```python
from build123d import *

# Parameters (mm, degrees)
F0_R     = 1
F1_DEPTH = 75
F2_W     = 65
F2_H     = 95
F3_DEPTH = 63
F4_R     = 1.7
F5_DEPTH = 7.001
F6_R     = 4


with BuildPart() as f1:
    # F0 (on Right) → F1 (new body)
    with BuildSketch(Plane.YZ):
        with BuildLine():
            Line((0, 72), (0, 0))
            Line((0, 0), (50, 0))
            ThreePointArc((50, 0), (64.142136, 5.857864), (70, 20))
            Line((70, 20), (70, 69))
            ThreePointArc((70, 69), (69.12132, 71.12132), (67, 72))
            Line((67, 72), (60.95857, 72))
            ThreePointArc((60.95857, 72), (57.269006, 70.731503), (55.139509, 67.462372))
            Line((55.139509, 67.462372), (50.118783, 47.483938))
            ThreePointArc((50.118783, 47.483938), (49.969332, 46.149869), (50.180201, 44.824121))
            Line((50.180201, 44.824121), (53.069629, 35.224997))
            ThreePointArc((53.069629, 35.224997), (50.230854, 29.932138), (44.933914, 32.763293))
            Line((44.933914, 32.763293), (41.069777, 45.467928))
            ThreePointArc((41.069777, 45.467928), (40.854911, 46.800259), (41.00419, 48.141522))
            Line((41.00419, 48.141522), (45.437209, 65.781356))
            ThreePointArc((45.437209, 65.781356), (44.530911, 70.074637), (40.587992, 72))
            Line((40.587992, 72), (0, 72))
        make_face()
        with Locations((66, 68)):
            Circle(F0_R, mode=Mode.SUBTRACT)
    extrude(amount=F1_DEPTH)

    # F2 (on face) → F3 (cut)
    with BuildSketch(Plane(origin=(0, 70, 0), x_dir=(-1, 0, 0), z_dir=(0, 1, 0))):
        with Locations((-37.5, 41.631669)):
            Rectangle(F2_W, F2_H)
    extrude(amount=-F3_DEPTH, mode=Mode.SUBTRACT)

    # F4 (on face) → F5 (cut, through all)
    with BuildSketch(Plane(origin=(0, 7, 0), x_dir=(-1, 0, 0), z_dir=(0, 1, 0))):
        with Locations((-61.5, 60)):
            Circle(F4_R)
        with Locations((-61.5, 12)):
            Circle(F4_R)
        with Locations((-13.5, 12)):
            Circle(F4_R)
        with Locations((-13.5, 60)):
            Circle(F4_R)
        with Locations((-37.5, 52)):
            Circle(F4_R)
        with Locations((-37.5, 20)):
            Circle(F4_R)
    extrude(amount=-F5_DEPTH, mode=Mode.SUBTRACT)

    # F6
    f6_edges = [f1.edges().sort_by_distance(p)[0] for p in [
        (70, 7, 36),
        (5, 7, 36),
    ]]
    fillet(f6_edges, radius=F6_R)


solid = f1.part
```
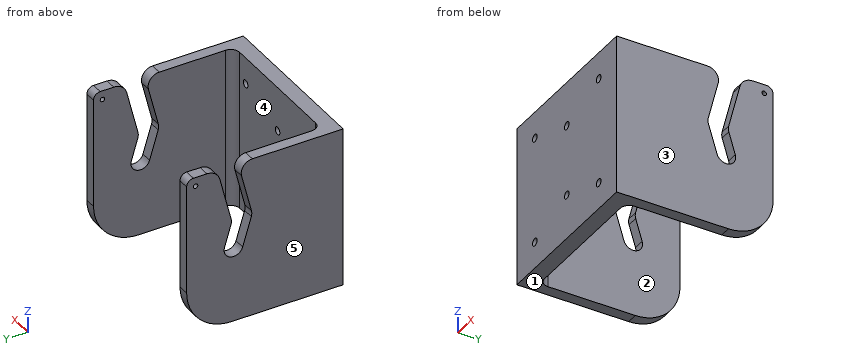
Work out the finished part from the listing and answer in its coordinate system (mm). Face numbers are marked on the shaded views. A direction names the side the tool comes from. Give positions to 0.01 mm unless a question says otherwise; leave off trailing zeros. Write each loop counter-clockwise with the first axis right and the second up, starting at its lowest first coordinate (ties: lowest second). Pieces come first, ordered by that corner, then holes.
(1) Which of the six approach directions +Z, -Z, +X, -X, +Y, -Y give full straight-line access (tool end or side, diameter ignored) to the marked faces 1 and 2?
Final values:
face 1: -Z, +X, -X, +Y, -Y
face 2: +Z, -Z, +Y
(2) The part is cut by section A-A on y = 20. Write down the section's boundary in (x, z).
Final values:
outline: (0, 0) - (5, 0) - (5, 72) - (0, 72) - close; (70, 0) - (75, 0) - (75, 72) - (70, 72) - close
(3) The part is cut by section D-D on z = 34. Write down the section's boundary in (x, y), plus the area to 3 significant figures.
Final values:
outline: (0, 0) - (75, 0) - (75, 44.56) - (70, 44.56) - (70, 11) arc R4 cw to (66, 7) - (9, 7) arc R4 cw to (5, 11) - (5, 44.56) - (0, 44.56) - close; (0, 53.25) - (5, 53.25) - (5, 70) - (0, 70) - close; (70, 53.25) - (75, 53.25) - (75, 70) - (70, 70) - close
area: 1,070 mm2
(4) The part is cut by section C-C on z = 23.5. Write down the section's boundary in (x, y).
Final values:
outline: (0, 0) - (75, 0) - (75, 70) - (70, 70) - (70, 11) arc R4 cw to (66, 7) - (9, 7) arc R4 cw to (5, 11) - (5, 70) - (0, 70) - close
(5) The part is cut by section B-B on x = 37.5. Write down the section's boundary in (y, z).
Final values:
outline: (0, 0) - (7, 0) - (7, 18.3) - (0, 18.3) - close; (0, 21.7) - (7, 21.7) - (7, 50.3) - (0, 50.3) - close; (0, 53.7) - (7, 53.7) - (7, 72) - (0, 72) - close
(6) Straight lines are drawn through the part: line 1 (Z direction, x = 13.5, y = 4.25); line 2 (X direction, y = 45, z = 11); line 3 (Z direction, x = 37.5, y = 3.5). For each, find the intervals that lie inside material, in ascending order.
Final values:
line 1: z = 0 to 10.3, 13.7 to 58.3, 61.7 to 72
line 2: x = 0 to 5, 70 to 75
line 3: z = 0 to 18.3, 21.7 to 50.3, 53.7 to 72
(7) Flat-ended cylindrical pins translate along their axes: pin 1 Ø2 at (x, z) = (13.5, 12) entering from -Y; pin 2 Ø17 at (x, z) = (45.5, 39) entering from +Y. Find the tip coordinate at first contact, or state that the pin passes through.
Final values:
pin 1: passes through
pin 2: stops at y = 7
(8) The mould has two halves that part along X. Classify the marked faces 3, 4 and 5: pulls with the +X half, pulls with the -X half, needs draft (parallel to the pull), parting line crosses it, or undercut.
Final values:
face 3: pulls with the +X half
face 4: undercut
face 5: pulls with the -X half
